Design review of the part built by this model. Coordinates are the model's own, in mm. A direction names the side the tool comes from. Round coordinates to 2 decimals unless told otherwise and drop trailing zeros. Order: outer loops, then holes, each group sorted by start corner. A loop starts at its lowest first (then second) coordinate and runs counter-clockwise, first axis right, second up.
from build123d import *

# Parameters (mm, degrees)
SKETCH1_W           = 38.1
SKETCH1_H           = 50.8
BOSS_EXTRUDE1_DEPTH = 15.24
SKETCH2_W           = 17.78
SKETCH2_H           = 6.35
SKETCH2_W_2         = 15.24
CUT_EXTRUDE1_DEPTH  = 15.24
SKETCH3_R           = 4.7625
CUT_EXTRUDE2_DEPTH  = 45.45
FILLET1_R           = 2.54


with BuildPart() as part:
    # Sketch1 → Boss-Extrude1 (new body)
    with BuildSketch(Plane(origin=(0, 0, 0), x_dir=(1, 0, 0), z_dir=(0, 1, 0))):
        Rectangle(SKETCH1_W, SKETCH1_H)
    extrude(amount=BOSS_EXTRUDE1_DEPTH)

    # Sketch2 → Cut-Extrude1 (cut)
    with BuildSketch(Plane(origin=(0, 15.24, 0), x_dir=(1, 0, 0), z_dir=(0, 1, 0))):
        with Locations((-10.16, 22.225)):
            Rectangle(SKETCH2_W, SKETCH2_H)
        with Locations((11.43, 22.225)):
            Rectangle(SKETCH2_W_2, SKETCH2_H)
        with Locations((-10.16, -22.225)):
            Rectangle(SKETCH2_W, SKETCH2_H)
        with Locations((11.43, -22.225)):
            Rectangle(SKETCH2_W_2, SKETCH2_H)
        Polygon((0, -25.4), (-1.27, -19.05), (-1.27, -25.4), align=None)
        Polygon((0, 25.4), (-1.27, 25.4), (-1.27, 19.05), align=None)
    extrude(amount=-CUT_EXTRUDE1_DEPTH, mode=Mode.SUBTRACT)

    # Sketch3 → Cut-Extrude2 (cut, through all)
    with BuildSketch(Plane.XY.offset(19.05)):
        with BuildLine():
            ThreePointArc((-19.05, 7.62), (-16.818153673, 13.008153673), (-11.43, 15.24))
            Line((-11.43, 15.24), (-19.05, 15.24))
            Line((-19.05, 15.24), (-19.05, 7.62))
        make_face()
        with BuildLine():
            ThreePointArc((-11.43, 0), (-16.818153673, 2.231846327), (-19.05, 7.62))
            Line((-19.05, 7.62), (-19.05, 0))
            Line((-19.05, 0), (-11.43, 0))
        make_face()
        with Locations((-11.43, 7.62)):
            Circle(SKETCH3_R)
    extrude(amount=-CUT_EXTRUDE2_DEPTH, mode=Mode.SUBTRACT)

    # Fillet1
    fillet1_edges = [part.edges().sort_by_distance(p)[0] for p in [
        (11.43, 15.24, 19.05),
        (11.43, 0, 19.05),
        (11.43, 0, -19.05),
        (11.43, 15.24, -19.05),
    ]]
    fillet(fillet1_edges, radius=FILLET1_R)


solid = part.part
1) To check wall thickness, follow line 1 along Y through (x, z) = (-11.43, -9); line 2 along Z through (x, y) = (-16, 13.25); line 3 along X through (y, z) = (4, -3.5). State the ranges of each line that lie inside material, in increasing order.
Results:
line 1: y = 0 to 2.86, 12.38 to 15.24
line 2: z = -19.05 to 19.05
line 3: x = -18.14 to -14.52, -8.34 to 19.05
2) Take a section at C-C on x = -15. Give the boundary of the cut face in (y, z), plus the area to 3 significant figures.
Results:
outline: (0.89, -19.05) - (4.47, -19.05) - (4.47, 19.05) - (0.89, 19.05) - close; (10.77, -19.05) - (14.35, -19.05) - (14.35, 19.05) - (10.77, 19.05) - close
area: 273 mm2
3) For faces 4 (the face through (11.537, 0.724, 18.286)), 5 (the face through (11.5, 14.5, 18.3)), 6 (the face through (-6, 8, 19.05)), list the 3-axis set-ups (+Z, -Z, +X, -X, +Y, -Y) from which the entire face can be reached by the end or side of a thin tool; tool diameter is ignored.
Results:
face 4: +Z, +X, -Y
face 5: +Z, +X, +Y
face 6: +Z, -X, +Y, -Y
4) Clearance check with flat-ended pins moving along their axes: P1, Ø3, axis at x = -6.5, y = 4.5, coming from the +Z side; P2, Ø1, axis at y = 3, z = 7, coming from the -X side; P3, Ø8.5, axis at x = -11.43, y = 7.62, coming from the -Z side; P4, Ø7.5, axis at x = -9.5, y = 8.5, coming from the -Z side. State where each tip first meets the part, or that it passes through.
Results:
P1: stops at z = 19.05
P2: stops at x = -17.84
P3: passes through
P4: stops at z = -19.05
5) Take a section at B-B on y = 5. Give the boundary of the cut face in (x, z), plus the area to 3 significant figures.
Results:
outline: (-18.59, -19.05) - (-15.41, -19.05) - (-15.41, 19.05) - (-18.59, 19.05) - close; (-7.45, -19.05) - (-1.27, -19.05) - (0, -25.4) - (3.81, -25.4) - (3.81, -19.05) - (19.05, -19.05) - (19.05, 19.05) - (3.81, 19.05) - (3.81, 25.4) - (0, 25.4) - (-1.27, 19.05) - (-7.45, 19.05) - close
area: 1,190 mm2
6) Take a section at D-D on x = 6.5. Give the boundary of the cut face in (y, z).
Results:
outline: (0, -16.51) arc R2.54 ccw to (2.54, -19.05) - (12.7, -19.05) arc R2.54 ccw to (15.24, -16.51) - (15.24, 16.51) arc R2.54 ccw to (12.7, 19.05) - (2.54, 19.05) arc R2.54 ccw to (0, 16.51) - close
7) The part is to be moulded in two halves that separate along Y. For faces 1 (the face through (-16.188, 7.829, 0.267)), 2 (the face through (2, 8, 25.4)), 3 (the face through (11.5, 14.5, -18.3)), say which applies: released by +Y, released by -Y, zero draft, split by the parting line, or undercut.
Results:
face 1: undercut
face 2: zero draft
face 3: released by +Y
